Input: part model. Units: mm. Frame: model coordinates. A direction names the side the tool comes from. Round coordinates to 2 decimals unless told otherwise and drop trailing zeros. Write each loop counter-clockwise with the first axis right and the second up, starting at its lowest first coordinate (ties: lowest second). Pieces come first, ordered by that corner, then holes. Notation, with made-up numbers: (77, -31.5) - (93, -31.5) arc R31 ccw to (93, 0.5) - close; hole circle Ø6 at (70.25, 20.5). An arc over 180 degrees is marked (long way). Use one line per item in the form item = value.
```python
from build123d import *

# Parameters (mm, degrees)
F0_R     = 19
F0_R_2   = 1.25
F0_R_3   = 6.5
F1_DEPTH = 65
F2_DEPTH = 5
F3_R     = 1.6
F4_DEPTH = 12
F5_R     = 5
F5_R_2   = 1.6
F6_DEPTH = 10


with BuildPart() as f1:
    # F0 (on Front) → F1 (new body)
    with BuildSketch(Plane.XZ):
        Circle(F0_R)
        with Locations((-12.5, 0)):
            Circle(F0_R_2, mode=Mode.SUBTRACT)
        Circle(F0_R_3, mode=Mode.SUBTRACT)
        with Locations((12.5, 0)):
            Circle(F0_R_2, mode=Mode.SUBTRACT)
        Circle(F0_R_3)
    extrude(amount=-F1_DEPTH)

    # F0 (on Front) → F2 (join)
    with BuildSketch(Plane.XZ):
        Circle(F0_R_3)
    extrude(amount=F2_DEPTH)

    # F3 (on face) → F4 (join)
    with BuildSketch(Plane.XZ.offset(5)):
        Circle(F3_R)
    extrude(amount=F4_DEPTH)

    # F5 (on face) → F6 (join)
    with BuildSketch(Plane.XZ.offset(17)):
        Circle(F5_R)
        Circle(F5_R_2, mode=Mode.SUBTRACT)
    extrude(amount=-F6_DEPTH)


solid = f1.part
```
(1) Draft query along Z for faces 1 (the face through (0, -17, 0)), 2 (the face through (-13.75, 32.04, 0.05)), 3 (the face through (-1.27, -5.99, -0.97)). Return one class per face: released by +Z, released by -Z, zero draft, split by the parting line, or undercut.
Derived:
face_1 = zero draft
face_2 = undercut
face_3 = split by the parting line
(2) Cut plane C-C on x = 0. Output: boundary loops of the cut face in (y, z).
Derived:
outline = (-17, -5) - (-7, -5) - (-7, -1.6) - (-5, -1.6) - (-5, -6.5) - (0, -6.5) - (0, -19) - (65, -19) - (65, 19) - (0, 19) - (0, 6.5) - (-5, 6.5) - (-5, 1.6) - (-7, 1.6) - (-7, 5) - (-17, 5) - close
(3) Cut plane A-A on x = -12.5. Output: boundary loops of the cut face in (y, z), then the cut area to 3 significant figures.
Derived:
outline = (0, -14.31) - (65, -14.31) - (65, -1.25) - (0, -1.25) - close; (0, 1.25) - (65, 1.25) - (65, 14.31) - (0, 14.31) - close
area = 1,700 mm^2
(4) Cut plane D-D on y = 7. Output: boundary loops of the cut face in (x, z).
Derived:
outline = circle Ø38 at (0, 0); hole circle Ø2.5 at (-12.5, 0); hole circle Ø2.5 at (12.5, 0)
(5) Access query for faces 4 (the face through (8.767, 32.045, -16.856)), 5 (the face through (1.4, -5, -1.4)), 6 (the face through (-5.158, -2.465, -3.955)). Directions: +Z, -Z, +X, -X, +Y, -Y. A direction counts if a zero-diameter tool reaches every point of the face in a straight line with its end or side. Return the directions, or none.
Derived:
face_4 = +Y, -Y
face_5 = none
face_6 = -Y
(6) Material intervals for L1, parallel to Y at x = 8, z = -4.5; L2, parallel to Z at x = 12.5, y = 17; L3, parallel to Y at x = -0.5, z = 5.5, sorted ascending.
Derived:
L1 = 0 to 65
L2 = -14.31 to -1.25, 1.25 to 14.31
L3 = -5 to 65
(7) First-contact query: pin 1 Ø3 at (x, y) = (-1, 41.5) entering from -Z; pin 2 Ø5 at (y, z) = (12.5, 8.5) entering from -X; pin 3 Ø12 at (x, y) = (10, 32.5) entering from -Z; pin 4 Ø12 at (x, z) = (2.5, 8) entering from -Y. Flat tips, straight axial feed; report the tip coordinate or a pass-through.
Derived:
pin_1 = -19
pin_2 = -18.03
pin_3 = -18.57
pin_4 = -17
(8) Cut plane B-B on z = -3.5. Output: boundary loops of the cut face in (x, y).
Derived:
outline = (-18.67, 0) - (-5.48, 0) - (-5.48, -5) - (5.48, -5) - (5.48, 0) - (18.67, 0) - (18.67, 65) - (-18.67, 65) - close; (-3.57, -17) - (3.57, -17) - (3.57, -7) - (-3.57, -7) - close
